The model under review builds one solid part; all positions refer to its coordinate system, in mm. A direction names the side the tool comes from. Round coordinates to 2 decimals unless told otherwise and drop trailing zeros. Write each loop counter-clockwise with the first axis right and the second up, starting at its lowest first coordinate (ties: lowest second). Pieces come first, ordered by that corner, then holes. Notation, with made-up numbers: M 33,40.25 L 84,40.25 A32 ccw 84,70.25 Z; hole C 21,-17 d5. An arc over 180 degrees is marked long. One line per item, written item: value. Start each with the question number.
1) Take a section at D-D, the plane z = -2.75. Write out the cut boundary in (x, y), and give its area (3 significant figures).
2) Tool access review of faces 4 (the face through (-3.338, 15.034, -4.93)), 5 (the face through (4, 0, 3)): name each direction out of +Z, -Z, +X, -X, +Y, -Y from which nothing blocks a thin tool from reaching the whole face with its end or side.
3) For P1, Ø3, axis at y = 6.5, z = -7.5, coming from the -X side; P2, Ø3, axis at x = -12, z = -3.5, coming from the +Y side; P3, Ø2, axis at x = 13.5, y = 11, coming from the +Z side; P4, Ø1, axis at x = 1.5, z = -7, coming from the +Y side, all flat-tipped, find the tip position at first contact; note any pin that passes through.
4) Take a section at A-A, the plane x = 0. Write out the cut boundary in (y, z), and give its area (3 significant figures).
5) Mouldability with a two-part tool opening along X and no side actions: class faces 1 (the face through (9.139, 14.334, 1.479)), 2 (the face through (0, -4, -10)), 3 (the face through (-2.539, -1.947, -3.409)) as +X half, -X half, draft (parallel to the pull), parting line (faces both ways), or undercut.
6) Take a section at C-C, the plane x = 15. Write out the cut boundary in (y, z), and give its area (3 significant figures).
7) Wall thickness on probe 1 along Y at (x, z) = (0, -3.5); probe 2 along X at (y, z) = (2.5, -5); probe 3 along X at (y, z) = (-0.5, 2): over which ranges is each line inside the solid? List them lowest first.
from build123d import *

# Parameters (mm, degrees)
SKETCH_R     = 17
PAD_DEPTH    = 3
SKETCH001_R  = 15.4
PAD001_DEPTH = 10
SKETCH002_R  = 3.2
POCKET_DEPTH = 13.001


with BuildPart() as part:
    # Sketch → Pad (new body)
    with BuildSketch(Plane.XY):
        Circle(SKETCH_R)
    extrude(amount=PAD_DEPTH)

    # Sketch001 (on Face2 of Pad) → Pad001 (join)
    with BuildSketch(Plane(origin=(0, 0, 0), x_dir=(1, 0, 0), z_dir=(0, 0, -1))):
        Circle(SKETCH001_R)
    extrude(amount=PAD001_DEPTH)

    # Sketch002 → Pocket (cut, through all)
    with BuildSketch(Plane.XY.offset(3)):
        Circle(SKETCH002_R)
    extrude(amount=-POCKET_DEPTH, mode=Mode.SUBTRACT)


solid = part.part
Checked values:
1. outline: C 0,0 d30.8; hole C 0,0 d6.4
1. area: 713 mm2
2. face 4: -Z
2. face 5: +Z, +X, -X, +Y, -Y
3. P1: stops at x = -14.57
3. P2: stops at y = 11.27
3. P3: stops at z = 3
3. P4: stops at y = 15.37
4. outline: M -17,0 L -15.4,0 L -15.4,-10 L -3.2,-10 L -3.2,3 L -17,3 Z; M 3.2,-10 L 15.4,-10 L 15.4,0 L 17,0 L 17,3 L 3.2,3 Z
4. area: 327 mm2
5. face 1: parting line
5. face 2: draft
5. face 3: undercut
6. outline: M -8,0 L -3.49,0 L -3.49,-10 L 3.49,-10 L 3.49,0 L 8,0 L 8,3 L -8,3 Z
6. area: 118 mm2
7. probe 1: y = -15.4 to -3.2, 3.2 to 15.4
7. probe 2: x = -15.2 to -2, 2 to 15.2
7. probe 3: x = -16.99 to -3.16, 3.16 to 16.99
